Design review of the part built by this model. Coordinates are the model's own, in mm. Round coordinates to 2 decimals unless told otherwise and drop trailing zeros. Write each loop counter-clockwise with the first axis right and the second up, starting at its lowest first coordinate (ties: lowest second). Pieces come first, ordered by that corner, then holes. Notation, with made-up numbers: M 16,47.25 L 37,47.25 A29 ccw 37,76.25 Z; hole C 52.25,-25.5 d9. An arc over 180 degrees is marked long. One line per question, with ' | ' between items. Start each with the question number.
Item 1: Add section B-B, the plane x = 163. State the section outline as (y, z) points.
Item 2: Add section A-A, the plane y = 1.55. State the section outline as (x, z) points.
Item 3: Insertion check: pin 1 Ø1.5 at (y, z) = (2, -28) entering from -X; pin 2 Ø1 at (x, y) = (118.5, 2.5) entering from -Z; pin 3 Ø0.9 at (x, y) = (178.5, 2) entering from +Z. Each pin has a flat end and moves straight along its axis. Give the tip position at first contact, or say it passes through.
Item 4: For L1, parallel to Z at x = 19, y = 0.1; L2, parallel to Z at x = 107, y = 2.85, list the stretches that pass through material, from the lowest coordinate up.
```python
from build123d import *

# Parameters (mm, degrees)
SKETCH_1_W      = 10
SKETCH_1_H      = 10
EXTRUDE_1_DEPTH = 3


with BuildPart() as part:
    # 草图1 → 凸台-拉伸1 (new body)
    with BuildSketch(Plane(origin=(0, 0, 0), x_dir=(1, 0, 0), z_dir=(0, 1, 0))):
        Polygon((160, -3), (180, -3), (180, 0), (180, 27), (175, 27), (175, 30), (180, 30), (180, 230), (180, 233), (175, 233), (175, 230), (5, 230), (5, 233), (0, 233), (0, 230), (0, 30), (5, 30), (5, 27), (0, 27), (0, 0), (0, -3), (20, -3), (20, -6), (160, -6), align=None)
        with Locations((90, 12)):
            Rectangle(SKETCH_1_W, SKETCH_1_H, mode=Mode.SUBTRACT)
    extrude(amount=EXTRUDE_1_DEPTH)


solid = part.part
```
Computed values:
1) outline: M 0,-230 L 3,-230 L 3,3 L 0,3 Z
2) outline: M 0,-233 L 5,-233 L 5,-230 L 175,-230 L 175,-233 L 180,-233 L 180,-30 L 175,-30 L 175,-27 L 180,-27 L 180,3 L 160,3 L 160,6 L 20,6 L 20,3 L 0,3 L 0,-27 L 5,-27 L 5,-30 L 0,-30 Z; hole M 85,-17 L 95,-17 L 95,-7 L 85,-7 Z
3) pin 1: stops at x = 5 | pin 2: stops at z = -230 | pin 3: stops at z = 3
4) L1: z = -230 to 3 | L2: z = -230 to 6
